Can you work these out from the model? Positions are in its coordinate system, mm. Face numbers are marked on the shaded views. A direction names the side the tool comes from. Round coordinates to 2 decimals unless told otherwise and drop trailing zeros. Order: outer loops, then holes, each group sorted by start corner. A loop starts at its lowest first (then second) coordinate and runs counter-clockwise, first axis right, second up. Notation, with made-up numbers: M -22,53 L 29,53 A24 cw 29,68 Z; hole C -11,51.25 d2. An arc over 180 degrees is marked long. Answer as a JSON object with one key per item and string values. Group by question number.
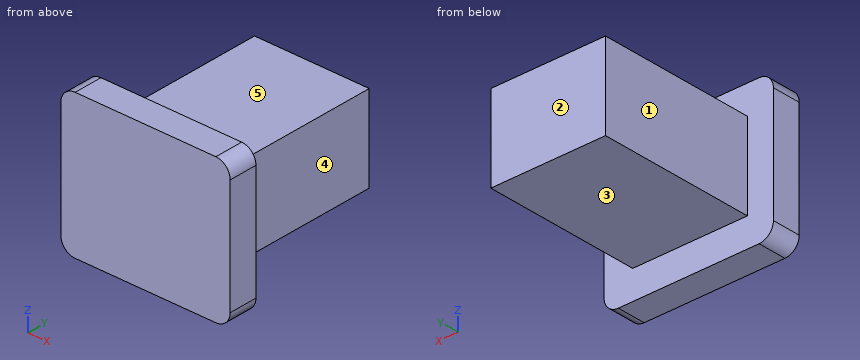
```python
from build123d import *

# Parameters (mm, degrees)
F1_DEPTH = 10
F2_W     = 40
F2_H     = 30
F3_DEPTH = 55


with BuildPart() as f1:
    # F0 (on Front) → F1 (new body)
    with BuildSketch(Plane.XZ):
        with BuildLine():
            Line((25.653138, 14.966757), (-23.414218, 14.966757))
            ThreePointArc((-23.414218, 14.966757), (-26.949752, 13.502291), (-28.414218, 9.966757))
            Line((-28.414218, 9.966757), (-28.414218, -30.033243))
            ThreePointArc((-28.414218, -30.033243), (-26.949752, -33.568777), (-23.414218, -35.033243))
            Line((-23.414218, -35.033243), (25.653138, -35.033243))
            ThreePointArc((25.653138, -35.033243), (29.188672, -33.568777), (30.653138, -30.033243))
            Line((30.653138, -30.033243), (30.653138, 9.966757))
            ThreePointArc((30.653138, 9.966757), (29.188672, 13.502291), (25.653138, 14.966757))
        make_face()
    extrude(amount=F1_DEPTH)

    # F2 (on Front) → F3 (join)
    with BuildSketch(Plane.XZ):
        with Locations((0.653138, -10.033243)):
            Rectangle(F2_W, F2_H)
    extrude(amount=-F3_DEPTH)


solid = f1.part
```
1) If we section it at C-C on y = 18.5: Write out the boundary of the cut face in (x, z), plus the area to 3 significant figures.
2) If we section it at A-A on x = -18: Write out the boundary of the cut face in (y, z), plus the area to 3 significant figures.
3) For pin 1 (4 mm diameter, centred on y = 7.5, z = 6, fed in from -X); pin 2 (20 mm diameter, centred on x = -5, y = 37, fed in from -Z); pin 3 (2 mm diameter, centred on x = -13.5, y = 15, fed in from +Z), each with a flat end and sliding along its axis, tell me the tip position at first contact or that it passes through.
4) If we section it at B-B on z = -10.5: Write out the boundary of the cut face in (x, y), plus the area to 3 significant figures.
5) If we section it at D-D on z = -29: Write out the boundary of the cut face in (x, y), plus the area to 3 significant figures.
6) I need wall thicknesses on line 1 along X through (y, z) = (13, -3); line 2 along Z through (x, y) = (-6.5, 22); line 3 along Y through (x, z) = (-25, -11). Which ranges of each line are inside material? Lowest first, please.
7) Which directions (+Z, -Z, +X, -X, +Y, -Y) give clear straight access to the entire face, cutting with the end or side of a thin tool? Please do the marked faces 1, 2, 3, 4 and 5.
Findings:
{
 "1": {"outline": "M -19.35,-25.03 L 20.65,-25.03 L 20.65,4.97 L -19.35,4.97 Z", "area": "1,200 mm^2"},
 "2": {"outline": "M -10,-35.03 L 0,-35.03 L 0,-25.03 L 55,-25.03 L 55,4.97 L 0,4.97 L 0,14.97 L -10,14.97 Z", "area": "2,150 mm^2"},
 "3": {"pin 1": "stops at x = -19.35", "pin 2": "stops at z = -25.03", "pin 3": "stops at z = 4.97"},
 "4": {"outline": "M -28.41,-10 L 30.65,-10 L 30.65,0 L 20.65,0 L 20.65,55 L -19.35,55 L -19.35,0 L -28.41,0 Z", "area": "2,790 mm^2"},
 "5": {"outline": "M -28.41,-10 L 30.65,-10 L 30.65,0 L -28.41,0 Z", "area": "591 mm^2"},
 "6": {"line 1": "x = -19.35 to 20.65", "line 2": "z = -25.03 to 4.97", "line 3": "y = -10 to 0"},
 "7": {"face 1": "+Z, -Z, -X, +Y", "face 2": "+Z, -Z, +X, -X, +Y", "face 3": "-Z, +X, -X, +Y", "face 4": "+Z, -Z, +X, +Y", "face 5": "+Z, +X, -X, +Y"}
}
